from build123d import *

# Parameters (mm, degrees)
F0_W     = 20
F0_H     = 60
F1_DEPTH = 25
F3_DEPTH = 180.001
F5_DEPTH = 25.001
F6_W     = 20
F6_H     = 10
F7_DEPTH = 25.001


with BuildPart() as f1:
    # F0 (on Front) → F1 (new body)
    with BuildSketch(Plane.XZ):
        Polygon((-46.595383, 21.920689), (-46.595383, 1.920689), (133.404617, 1.920689), (133.404617, 21.920689), (113.404617, 21.920689), (93.404617, 21.920689), (73.404617, 21.920689), (53.404617, 21.920689), (33.404617, 21.920689), (13.404617, 21.920689), (-6.595383, 21.920689), (-26.595383, 21.920689), align=None)
        with Locations((-36.595383, 51.920689)):
            Rectangle(F0_W, F0_H)
        with Locations((123.404617, 51.920689)):
            Rectangle(F0_W, F0_H)
        with Locations((3.404617, 51.920689)):
            Rectangle(F0_W, F0_H)
        with Locations((83.404617, 51.920689)):
            Rectangle(F0_W, F0_H)
        with Locations((43.404617, 51.920689)):
            Rectangle(F0_W, F0_H)
    extrude(amount=F1_DEPTH)

    # F2 (on face) → F3 (cut, through all)
    with BuildSketch(Plane.YZ.offset(133.404617)):
        Polygon((-18.75, 50.670689), (-18.75, 33.170689), (-12.5, 26.920689), (-6.25, 33.170689), (-6.25, 50.670689), (-12.5, 56.920689), align=None)
    extrude(amount=-F3_DEPTH, mode=Mode.SUBTRACT)

    # F4 (on face) → F5 (cut, through all)
    with BuildSketch(Plane.XZ.offset(25)):
        Polygon((-26.595383, 81.920689), (-46.595383, 81.920689), (-26.595383, 61.920689), align=None)
        Polygon((13.404617, 81.920689), (-6.595383, 81.920689), (13.404617, 61.920689), align=None)
        Polygon((53.404617, 81.920689), (33.404617, 81.920689), (53.404617, 61.920689), align=None)
        Polygon((93.404617, 81.920689), (73.404617, 81.920689), (93.404617, 61.920689), align=None)
        Polygon((133.404617, 81.920689), (113.404617, 81.920689), (133.404617, 61.920689), align=None)
    extrude(amount=-F5_DEPTH, mode=Mode.SUBTRACT)

    # F6 (on face) → F7 (cut, through all)
    with BuildSketch(Plane.XZ.offset(25)):
        with Locations((53.404617, 11.920689)):
            Rectangle(F6_W, F6_H)
    extrude(amount=-F7_DEPTH, mode=Mode.SUBTRACT)


solid = f1.part
The listing builds one solid part. Answer for the finished solid, in the listing's coordinates (mm). A direction names the side the tool comes from. Coordinates: 2 decimals unless noted, no trailing zeros. Write each loop counter-clockwise with the first axis right and the second up, starting at its lowest first coordinate (ties: lowest second). Pieces come first, ordered by that corner, then holes. Notation, with made-up numbers: M -14,88 L 25,88 A22 cw 25,111 Z; hole C 78.5,72 d5. An arc over 180 degrees is marked long. Put each result on its own line as item: value. Start each with the question number.
1. A cutting plane is placed at A-A on z = 60. Write down the section's boundary in (x, y), then the cut area to 3 significant figures.
2. A cutting plane is placed at D-D on z = 41. Count the separate pieces of the cut face and the enclosed holes in it, then the cut area to 3 significant figures.
3. Which of the six approach directions +Z, -Z, +X, -X, +Y, -Y give full straight-line access (tool end or side, diameter ignored) to faces 1 (the flat face through (123.54, -15.67, 30.09)), 2 (the flat face through (53, -13, 16.921)), 3 (the flat face through (53.405, -21, 42))?
4. Flat-ended cylindrical pins translate along their axes: P1, Ø5, axis at x = 79.5, y = -14.5, coming from the +Z side; P2, Ø8, axis at x = -25, z = 70.5, coming from the -Y side; P3, Ø2, axis at x = 50, y = -8.5, coming from the +Z side. Find the tip coordinate at first contact, or state that the pin passes through.
5. A cutting plane is placed at C-C on x = 46.5. Write down the section's boundary in (y, z), then the cut area to 3 significant figures.
6. Consider line 1 (X direction, y = -21.5, z = 43); line 2 (X direction, y = -13, z = 15); line 3 (X direction, y = -19.75, z = 67.5). Determine where each line is inside the solid, lowest interval first. Write a range as from..to.
7. A cutting plane is placed at B-B on y = -20.75. Write down the section's boundary in (x, z).
8. For a pull along Y with two mould halves and no side action, classify faces 4 (the flat face through (133.405, -12, 25)), 5 (the flat face through (42, 0, 34)), 6 (the flat face through (44, -6.25, 42)) as pulls with the +Y half, pulls with the -Y half, needs draft (parallel to the pull), parting line crosses it, or undercut.
Resolved:
1. outline: M -46.6,-25 L -26.6,-25 L -26.6,0 L -46.6,0 Z; M -6.6,-25 L 13.4,-25 L 13.4,0 L -6.6,0 Z; M 33.4,-25 L 53.4,-25 L 53.4,0 L 33.4,0 Z; M 73.4,-25 L 93.4,-25 L 93.4,0 L 73.4,0 Z; M 113.4,-25 L 133.4,-25 L 133.4,0 L 113.4,0 Z
1. area: 2,500 mm2
2. separate pieces: 10
2. enclosed holes: 0
2. area: 1,250 mm2
3. face 1: +X, -X
3. face 2: +Y, -Y
3. face 3: +Z, +Y, -Y
4. P1: stops at z = 78.33
4. P2: passes through
4. P3: stops at z = 66.33
5. outline: M -25,1.92 L 0,1.92 L 0,6.92 L -25,6.92 Z; M -25,16.92 L 0,16.92 L 0,68.83 L -25,68.83 Z; hole M -18.75,33.17 L -12.5,26.92 L -6.25,33.17 L -6.25,50.67 L -12.5,56.92 L -18.75,50.67 Z
5. area: 1,130 mm2
6. line 1: x = -46.6..-26.6, -6.6..13.4, 33.4..53.4, 73.4..93.4, 113.4..133.4
6. line 2: x = -46.6..43.4, 63.4..133.4
6. line 3: x = -46.6..-32.17, -6.6..7.83, 33.4..47.83, 73.4..87.83, 113.4..127.83
7. outline: M -46.6,1.92 L 133.4,1.92 L 133.4,61.92 L 113.4,81.92 L 113.4,21.92 L 93.4,21.92 L 93.4,61.92 L 73.4,81.92 L 73.4,21.92 L 53.4,21.92 L 53.4,61.92 L 33.4,81.92 L 33.4,21.92 L 13.4,21.92 L 13.4,61.92 L -6.6,81.92 L -6.6,21.92 L -26.6,21.92 L -26.6,61.92 L -46.6,81.92 Z; hole M 43.4,6.92 L 63.4,6.92 L 63.4,16.92 L 43.4,16.92 Z
8. face 4: needs draft
8. face 5: pulls with the +Y half
8. face 6: undercut
